CAD build for the part. Positions are in the model's coordinates, mm. Round coordinates to 2 decimals unless told otherwise and drop trailing zeros. Write each loop counter-clockwise with the first axis right and the second up, starting at its lowest first coordinate (ties: lowest second). Pieces come first, ordered by that corner, then holes. Notation, with made-up numbers: (53, -6.75) - (112, -6.75) arc R28 cw to (112, 16.25) - close; hole circle Ø1 at (-11, -9.5). An arc over 180 degrees is marked (long way). Answer in a Markdown table with one row per item.
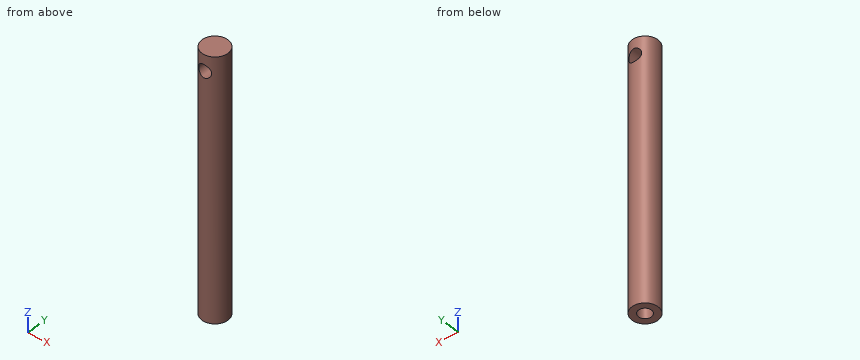
```python
from build123d import *

# Parameters (mm, degrees)
SKETCH_1_R               = 8
EXTRUDE_1_DEPTH          = 160
SKETCH_2_R               = 4
CUT_EXTRUDE_1_DEPTH      = 120
CUT_EXTRUDE_1_DEPTH_BACK = 120
SKETCH_3_R               = 4
CUT_EXTRUDE_2_DEPTH      = 10


with BuildPart() as part:
    # Sketch 1 → Extrude 1 (new body)
    with BuildSketch(Plane.XY):
        Circle(SKETCH_1_R)
    extrude(amount=EXTRUDE_1_DEPTH)

    # Sketch 2 → Cut-Extrude 1 (cut, two sides)
    with BuildSketch(Plane(origin=(0, 0, 0), x_dir=(1, 0, 0), z_dir=(0, 1, 0))) as cut_extrude_1_sk:
        with Locations((0, -150)):
            Circle(SKETCH_2_R)
    extrude(amount=CUT_EXTRUDE_1_DEPTH, mode=Mode.SUBTRACT)
    extrude(cut_extrude_1_sk.sketch, amount=-CUT_EXTRUDE_1_DEPTH_BACK, mode=Mode.SUBTRACT)

    # Sketch 3 → Cut-Extrude 2 (cut)
    with BuildSketch(Plane(origin=(0, 0, 0), x_dir=(-1, 0, 0), z_dir=(0, 0, -1))):
        Circle(SKETCH_3_R)
    extrude(amount=-CUT_EXTRUDE_2_DEPTH, mode=Mode.SUBTRACT)


solid = part.part
```
Q1. Saw through at C-C on z = 90. List the corners of the cut face in (x, y).
Computed:
| item | result |
|---|---|
| outline | circle Ø16 at (0, 0) |
Q2. Saw through at A-A on x = 0. List the corners of the cut face in (y, z).
Computed:
| item | result |
|---|---|
| outline | (-8, 0) - (-4, 0) - (-4, 10) - (4, 10) - (4, 0) - (8, 0) - (8, 146) - (-8, 146) - close; (-8, 154) - (8, 154) - (8, 160) - (-8, 160) - close |
Q3. Flat gauge pins, fed straight in: pin 1 (1 mm diameter, centred on y = 5, z = 35.5, fed in from -X); pin 2 (4 mm diameter, centred on x = 6, z = 117.5, fed in from +Y); pin 3 (5 mm diameter, centred on x = 0, y = 0, fed in from -Z). Where does each tip first touch, or does it go through?
Computed:
| item | result |
|---|---|
| pin 1 | stops at x = -6.61 |
| pin 2 | stops at y = 6.93 |
| pin 3 | stops at z = 10 |
Q4. Saw through at B-B on z = 150. List the corners of the cut face in (x, y).
Computed:
| item | result |
|---|---|
| outline | (-4, -6.93) - (-4, 6.93) arc R8 ccw to start; (4, -6.93) arc R8 ccw to (4, 6.93) - close |
Q5. Drill centre lines: line 1 (Y direction, x = 0, z = 5.25); line 2 (Z direction, x = -0.25, y = -3.75); line 3 (Y direction, x = 0.25, z = 37). Where is each one in solid material? Low to high.
Computed:
| item | result |
|---|---|
| line 1 | y = -8 to -4, 4 to 8 |
| line 2 | z = 10 to 146.01, 153.99 to 160 |
| line 3 | y = -8 to 8 |
Q6. Saw through at D-D on x = 5.75. List the corners of the cut face in (y, z).
Computed:
| item | result |
|---|---|
| outline | (-5.56, 0) - (5.56, 0) - (5.56, 160) - (-5.56, 160) - close |
